Geometry: final body of the model. Coordinates: model frame, mm. Face numbers are marked on the shaded views. A direction names the side the tool comes from. Coordinates: 2 decimals unless noted, no trailing zeros. Loops run counter-clockwise (first coordinate to the right, second up) from the corner with the lowest first, then second, coordinate; pieces in that order, holes last. Notation, with made-up numbers: (65.5, 36) -> (85.5, 36) arc R21 cw to (85.5, 54) -> close; hole circle Ø2 at (-2, 1.25). An arc over 180 degrees is marked (long way). One line per item, written item: value. Start each with the question number.
Item 1: Mould query, pull axis Y, two halves, no side actions, for the marked faces 3, 4 and 5. Classes: +Y half, -Y half, draft (parallel to the pull), parting line (faces both ways), or undercut.
Item 2: Set-up query: the marked faces 1 and 2. Return all of +Z, -Z, +X, -X, +Y, -Y with unobstructed straight access to the full face (end or side cutting, diameter ignored); none if empty.
Item 3: Contact query for flat-ended pins moving along their axis: pin 1 Ø1.9 at (x, y) = (3.81, 3.81) entering from -Z; pin 2 Ø4.5 at (x, y) = (1.5, 3) entering from -Z. Output: stop coordinate, or through.
Item 4: Section query A-A on y = -3.81. Return loops of the section in (x, z) (3 decimals), then the cut area to 3 significant figures.
Item 5: Ray query, probe 1 along Y at (x, z) = (-3.5, 1.75) (3 decimals); probe 2 along Y at (x, z) = (3.81, 9.2) (3 decimals). Return the intervals inside material, ascending. Write a range as from..to.
Item 6: Section query B-B on z = -0.25. Return loops of the section in (x, y) (3 decimals).
Item 7: Section query D-D on x = 0. Return loops of the section in (y, z) (3 decimals), then the cut area to 3 significant figures.
from build123d import *

# Parameters (mm, degrees)
F1_DEPTH = 9.525
F2_W     = 15.24
F2_H     = 15.24
F3_DEPTH = 20.32
F5_D     = 2.38125


with BuildPart() as f1:
    # F0 (on Front) → F1 (new body, symmetric)
    with BuildSketch(Plane.XZ):
        Polygon((9.525, 12.7), (-9.525, 12.7), (-9.525, -12.7), (9.525, -12.7), (9.525, 7.62), align=None)
    extrude(amount=F1_DEPTH, both=True)

    # F2 (on face) → F3 (cut)
    with BuildSketch(Plane(origin=(0, 0, -12.7), x_dir=(1, 0, 0), z_dir=(0, 0, -1))):
        Rectangle(F2_W, F2_H)
    extrude(amount=-F3_DEPTH, mode=Mode.SUBTRACT)

    # F5 (through all)
    with Locations(Plane(origin=(0, 0, 7.62), x_dir=(1, 0, 0), z_dir=(0, 0, -1))):
        with Locations((-3.81, 3.81), (3.81, -3.81)):
            Hole(F5_D / 2)


solid = f1.part
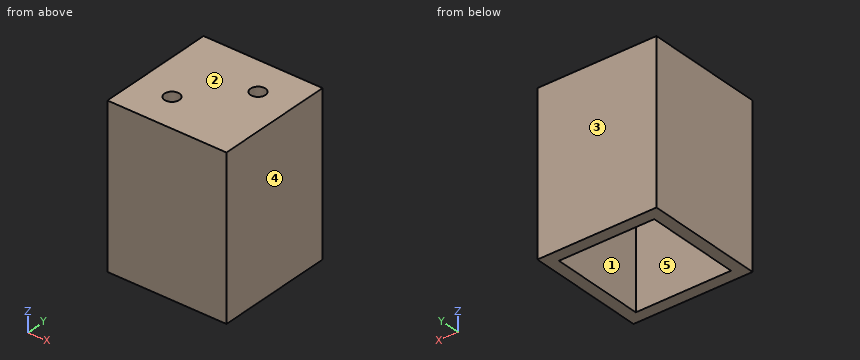
Reply:
1. face 3: +Y half
1. face 4: draft
1. face 5: undercut
2. face 1: -Z
2. face 2: +Z, +X, -X, +Y, -Y
3. pin 1: passes through
3. pin 2: stops at z = 7.62
4. outline: (-9.525, -12.7) -> (-7.62, -12.7) -> (-7.62, 7.62) -> (-5.001, 7.62) -> (-5.001, 12.7) -> (-9.525, 12.7) -> close; (-2.619, 7.62) -> (7.62, 7.62) -> (7.62, -12.7) -> (9.525, -12.7) -> (9.525, 12.7) -> (-2.619, 12.7) -> close
4. area: 162 mm²
5. probe 1: y = -9.525..-7.62, 7.62..9.525
5. probe 2: y = -9.525..2.619, 5.001..9.525
6. outline: (-9.525, -9.525) -> (9.525, -9.525) -> (9.525, 9.525) -> (-9.525, 9.525) -> close; hole (-7.62, -7.62) -> (7.62, -7.62) -> (7.62, 7.62) -> (-7.62, 7.62) -> close
7. outline: (-9.525, -12.7) -> (-7.62, -12.7) -> (-7.62, 7.62) -> (7.62, 7.62) -> (7.62, -12.7) -> (9.525, -12.7) -> (9.525, 12.7) -> (-9.525, 12.7) -> close
7. area: 174 mm²
